```python
from build123d import *

# Parameters (mm, degrees)
F1_DEPTH = 127
F3_R     = 4.7625
F4_DEPTH = 9.525
F6_R     = 4.7625
F7_DEPTH = 9.525
F8_R     = 4.7625
F9_DEPTH = 25.4


with BuildPart() as f1:
    # F0 (on Top) → F1 (new body)
    with BuildSketch(Plane.XY):
        Polygon((-355.6, 0), (-355.6, -9.525), (355.6, -9.525), (355.6, 0), (406.4, 0), (406.4, 9.525), (-406.4, 9.525), (-406.4, 0), align=None)
    extrude(amount=F1_DEPTH)

    # F3 (on offset) → F4 (join)
    with BuildSketch(Plane.YZ.offset(406.4)):
        with Locations((0, 63.5)):
            Circle(F3_R)
    extrude(amount=F4_DEPTH)

    # F6 (on offset) → F7 (join)
    with BuildSketch(Plane.YZ.offset(-406.4)):
        with Locations((0, 63.5)):
            Circle(F6_R)
    extrude(amount=-F7_DEPTH)

    # F8 (on Front) → F9 (cut)
    with BuildSketch(Plane.XZ):
        with Locations((396.875, 63.5)):
            Circle(F8_R)
        with Locations((-396.875, 63.5)):
            Circle(F8_R)
    extrude(amount=-F9_DEPTH, mode=Mode.SUBTRACT)


solid = f1.part
```
Source: CAD feature listing. Evaluate the final solid. Frame: model axes, mm. Coordinates: 2 decimals unless noted, no trailing zeros. Loops run counter-clockwise (first coordinate to the right, second up) from the corner with the lowest first, then second, coordinate; pieces in that order, holes last. Notation, with made-up numbers: M 12.5,-37 L 37.5,-37 A25 ccw 37.5,-7 Z; hole C 81.25,64.5 d6. An arc over 180 degrees is marked long. Use a Markdown table: item, result. Add a question column.
Q1. First-contact query: pin 1 (1 mm diameter, centred on y = 1, z = 106, fed in from +X); pin 2 (10.5 mm diameter, centred on y = 5, z = 76, fed in from -X); pin 3 (3 mm diameter, centred on y = -3.5, z = 73.5, fed in from +X). Flat tips, straight axial feed; report the tip coordinate or a pass-through.
Q2. Section query A-A, the plane z = 31. Return loops of the section in (x, y) (3 decimals).
Q3. Material intervals for L1, parallel to X at y = 7, z = 64; L2, parallel to X at y = 7.25, z = 27.5; L3, parallel to X at y = -2, z = 28, sorted ascending.
Result:
| question | item | result |
|---|---|---|
| 1 | pin 1 | stops at x = 406.4 |
| 1 | pin 2 | stops at x = -406.4 |
| 1 | pin 3 | stops at x = 355.6 |
| 2 | outline | M -406.4,0 L -355.6,0 L -355.6,-9.525 L 355.6,-9.525 L 355.6,0 L 406.4,0 L 406.4,9.525 L -406.4,9.525 Z |
| 3 | L1 | x = -406.4 to -401.61, -392.14 to 392.14, 401.61 to 406.4 |
| 3 | L2 | x = -406.4 to 406.4 |
| 3 | L3 | x = -355.6 to 355.6 |
